from build123d import *

# Parameters (mm, degrees)
SKETCH1_R             = 1.7907
BOSS_EXTRUDE1_DEPTH   = 3.6322
BOSS_EXTRUDE1_2_DEPTH = 3.6322
BOSS_EXTRUDE2_DEPTH   = 1.2446


with BuildPart() as part:
    # Sketch1 → Boss-Extrude1 (new body, symmetric)
    with BuildSketch(Plane.XY):
        with Locations((-4.7625, 0)):
            Circle(SKETCH1_R)
    extrude(amount=BOSS_EXTRUDE1_DEPTH, both=True)



with BuildPart() as body_2:
    # Sketch1 → Boss-Extrude1 2 (new body, symmetric)
    with BuildSketch(Plane.XY):
        with Locations((4.7625, 0)):
            Circle(SKETCH1_R)
    extrude(amount=BOSS_EXTRUDE1_2_DEPTH, both=True)


with BuildPart() as part_1:
    add(part.part)

    add(body_2.part)  # Boss-Extrude2 merges body 2
    # Sketch3 → Boss-Extrude2 (add)
    with BuildSketch(Plane.XY.offset(3.6322)):
        with BuildLine():
            ThreePointArc((-2.38125, 3.753354958), (-9.2075, 0), (-2.38125, -3.753354958))
            ThreePointArc((-2.38125, -3.753354958), (0, -3.061709915), (2.38125, -3.753354958))
            ThreePointArc((2.38125, -3.753354958), (9.2075, 0), (2.38125, 3.753354958))
            ThreePointArc((2.38125, 3.753354958), (0, 3.061709915), (-2.38125, 3.753354958))
        make_face()
    boss_extrude2 = extrude(amount=BOSS_EXTRUDE2_DEPTH)

    # Mirror1: Boss-Extrude2 across plane
    add(boss_extrude2.mirror(Plane.XY))


solid = part_1.part
Work out the finished part from the listing and answer in its coordinate system (mm). Give positions to 0.01 mm unless a question says otherwise; leave off trailing zeros. Loops run counter-clockwise (first coordinate to the right, second up) from the corner with the lowest first, then second, coordinate; pieces in that order, holes last. Notation, with made-up numbers: (5, 10) - (41, 10) arc R21 cw to (41, 42) - close; hole circle Ø3 at (-3.5, -8.75). An arc over 180 degrees is marked (long way). Answer in a Markdown table with one row per item. Add a question column.
Q1. Consider line 1 along Z through (x, y) = (-6.5, -2.5); line 2 along X through (y, z) = (0.5, -2.5); line 3 along X through (y, z) = (1, 2.25). Determine where each line is inside the solid, lowest interval first.
Q2. The part is cut by section B-B (y = 0). Determine the outline of the cut face in (x, z), and give its area (3 significant figures).
Q3. Each of these flat-tipped pins is pushed along its axis until it touches: P1, Ø4, axis at y = -3, z = -2.5, coming from the +X side; P2, Ø1, axis at y = -3, z = 2.5, coming from the -X side. Where does it stop, or does it pass through?
Q4. The part is cut by section C-C (z = -3.25). Determine the outline of the cut face in (x, y).
Q5. The part is cut by section D-D (y = -3.5). Determine the outline of the cut face in (x, z), and give its area (3 significant figures).
Q6. Determine the mould class of faces 1 (the flat face through (0, 0, 3.632)), 2 (the flat face through (0, 0, -4.877)), 3 (the flat face through (0, 0, 4.877)) for opening direction Z: released by +Z, released by -Z, zero draft, split by the parting line, or undercut.
Q7. The part is cut by section A-A (y = 3.25). Determine the outline of the cut face in (x, z), and give its area (3 significant figures).
Solution:
| question | item | result |
|---|---|---|
| 1 | line 1 | z = -4.88 to -3.63, 3.63 to 4.88 |
| 1 | line 2 | x = -6.48 to -3.04, 3.04 to 6.48 |
| 1 | line 3 | x = -6.25 to -3.28, 3.28 to 6.25 |
| 2 | outline | (-9.21, -4.88) - (9.21, -4.88) - (9.21, -3.63) - (6.55, -3.63) - (6.55, 3.63) - (9.21, 3.63) - (9.21, 4.88) - (-9.21, 4.88) - (-9.21, 3.63) - (-6.55, 3.63) - (-6.55, -3.63) - (-9.21, -3.63) - close; hole (-2.97, -3.63) - (2.97, -3.63) - (2.97, 3.63) - (-2.97, 3.63) - close |
| 2 | area | 97.9 mm² |
| 3 | P1 | stops at x = 9 |
| 3 | P2 | passes through |
| 4 | outline | circle Ø3.58 at (-4.76, 0); circle Ø3.58 at (4.76, 0) |
| 5 | outline | (-7.5, -4.88) - (-1.92, -4.88) - (-1.92, -3.63) - (-7.5, -3.63) - close; (-7.5, 3.63) - (-1.92, 3.63) - (-1.92, 4.88) - (-7.5, 4.88) - close; (1.92, -4.88) - (7.5, -4.88) - (7.5, -3.63) - (1.92, -3.63) - close; (1.92, 3.63) - (7.5, 3.63) - (7.5, 4.88) - (1.92, 4.88) - close |
| 5 | area | 27.8 mm² |
| 6 | face 1 | undercut |
| 6 | face 2 | released by -Z |
| 6 | face 3 | released by +Z |
| 7 | outline | (-7.79, -4.88) - (-1.28, -4.88) - (-1.28, -3.63) - (-7.79, -3.63) - close; (-7.79, 3.63) - (-1.28, 3.63) - (-1.28, 4.88) - (-7.79, 4.88) - close; (1.28, -4.88) - (7.79, -4.88) - (7.79, -3.63) - (1.28, -3.63) - close; (1.28, 3.63) - (7.79, 3.63) - (7.79, 4.88) - (1.28, 4.88) - close |
| 7 | area | 32.4 mm² |
